For this review, take the finished solid that the model builds, in its own axes (mm). A direction names the side the tool comes from. Coordinates: 2 decimals unless noted, no trailing zeros.
1. Mouldability with a two-part tool opening along X and no side actions: class faces 1 (the face through (27.623, -72, 19)), 2 (the face through (28, -75, 25)) as pulls with the +X half, pulls with the -X half, needs draft (parallel to the pull), parting line crosses it, or undercut.
2. Machinability: for faces 3 (the face through (25, -75.246, 19)), 4 (the face through (24, -64.946, 12)), 5 (the face through (26.273, -66, 19)), which of the approach directions +Z, -Z, +X, -X, +Y, -Y give a long, thin tool a straight path to every point of the face, cutting with its end or side? Answer none if there is none.
3. To check wall thickness, follow probe 1 along Z at (x, y) = (25.5, -68.75); probe 2 along X at (y, z) = (-71.75, 18); probe 3 along X at (y, z) = (-67, 24). State the ranges of each line that lie inside material, in increasing order.
4. Clearance check with flat-ended pins moving along their axes: P1, Ø0.9, axis at y = -67, z = 17.5, coming from the -X side; P2, Ø4, axis at x = 29, z = 2.5, coming from the -Y side; P3, Ø2, axis at y = -68, z = 19, coming from the -X side. State where each tip first meets the part, or that it passes through.
```python
from build123d import *

# Parameters (mm, degrees)
SALIENTE_EXTRUIR6_DEPTH = 25
CROQUIS10_W             = 3.1
CROQUIS10_H             = 12.5
CORTAR_EXTRUIR1_DEPTH   = 3
CROQUIS14_W             = 5.8
CROQUIS14_H             = 12.5
CORTAR_EXTRUIR3_DEPTH   = 7.3


with BuildPart() as part:
    # Croquis9 → Saliente-Extruir6 (new body)
    with BuildSketch(Plane.XY):
        with BuildLine():
            Line((5.43844596, -64.945905041), (44.007906752, -64.945905041))
            add(Edge.make_bspline(
                [(5.43844596, -64.945905041), (24.723176356, -116.374476469), (44.007906752, -64.945905041)],
                knots=[5.402163981, 5.402163981, 5.402163981, 7.164206633, 7.164206633, 7.164206633], degree=2, weights=[1, 0.636363636, 1]))
        make_face()
    extrude(amount=SALIENTE_EXTRUIR6_DEPTH)

    # Croquis10 → Cortar-Extruir1 (cut)
    with BuildSketch(Plane(origin=(0, -64.945905041, 0), x_dir=(1, 0, 0), z_dir=(0, 1, 0))):
        with Locations((24.722906752, -18.75)):
            Rectangle(CROQUIS10_W, CROQUIS10_H)
    extrude(amount=-CORTAR_EXTRUIR1_DEPTH, mode=Mode.SUBTRACT)

    # Croquis14 → Cortar-Extruir3 (cut)
    with BuildSketch(Plane(origin=(0, -67.945905041, 0), x_dir=(1, 0, 0), z_dir=(0, 1, 0))):
        with Locations((24.722906752, -18.75)):
            Rectangle(CROQUIS14_W, CROQUIS14_H)
    extrude(amount=-CORTAR_EXTRUIR3_DEPTH, mode=Mode.SUBTRACT)


solid = part.part
```
Results list:
1. face 1: undercut
1. face 2: needs draft
2. face 3: +Z
2. face 4: +Z, -Z, +X, -X, +Y
2. face 5: +Z, +Y
3. probe 1: z = 0 to 12.5
3. probe 2: x = 8.48 to 21.82, 27.62 to 40.97
3. probe 3: x = 6.25 to 23.17, 26.27 to 43.2
4. P1: stops at x = 6.06
4. P2: stops at y = -84.72
4. P3: stops at x = 6.25
